from build123d import *

# Parameters (mm, degrees)
F0_W     = 50.8
F0_H     = 3.175
F1_DEPTH = 354.8
F2_R     = 2.6162
F2_R_2   = 3.175
F3_DEPTH = 3.176


with BuildPart() as f1:
    # F0 (on Front) → F1 (new body)
    with BuildSketch(Plane.XZ):
        Rectangle(F0_W, F0_H)
    extrude(amount=F1_DEPTH)

    # F2 (on face) → F3 (cut, through all)
    with BuildSketch(Plane.XY.offset(1.5875)):
        with Locations((0, -158.35)):
            Circle(F2_R)
        with Locations((0, -196.45)):
            Circle(F2_R)
        with Locations((-19.05, -329.4)):
            Circle(F2_R)
        with Locations((19.05, -329.4)):
            Circle(F2_R)
        with Locations((19.05, -25.4)):
            Circle(F2_R)
        with Locations((-19.05, -25.4)):
            Circle(F2_R)
        with Locations((-15.3416, -252.4)):
            Circle(F2_R)
        with Locations((15.3416, -252.4)):
            Circle(F2_R)
        with Locations((15.3416, -102.4)):
            Circle(F2_R)
        with Locations((-15.3416, -102.4)):
            Circle(F2_R)
        with Locations((0, -269.6254)):
            Circle(F2_R_2)
        with Locations((0, -85.1746)):
            Circle(F2_R_2)
    extrude(amount=-F3_DEPTH, mode=Mode.SUBTRACT)


solid = f1.part
Check sheet for the modelled part. Datum: model origin and axes. Units: mm. Coordinates: 2 decimals unless noted, no trailing zeros. Write item = value, one per line. Start each with the question number.
1. Material ranges on line 1 (Y direction, x = -19.05, z = -0.15); line 2 (Y direction, x = 0, z = 0.6); line 3 (Y direction, x = 1, z = -0.7), recorded low to high.
2. Draft check along Y on faces 1 (the flat face through (0, -175, 1.588)), 2 (the cylindrical face through (-0.688, -88.274, 0.022)). Enter one of: released by +Y, released by -Y, zero draft, split by the parting line, or undercut.
3. Section check A-A on z = -1. Give the number of separate pieces and of enclosed holes in the cut face, then the cut area to 3 significant figures.
4. Depth check by flat-ended pin: P1, Ø4.5, axis at x = 15.34, y = -102.4, coming from the -Z side. Enter the tip coordinate at first touch or a pass-through.
Responses:
q1.line_1 = -354.8 to -332.02, -326.78 to -28.02, -22.78 to 0
q1.line_2 = -354.8 to -272.8, -266.45 to -199.07, -193.83 to -160.97, -155.73 to -88.35, -82 to 0
q1.line_3 = -354.8 to -272.64, -266.61 to -198.87, -194.03 to -160.77, -155.93 to -88.19, -82.16 to 0
q2.face_1 = zero draft
q2.face_2 = undercut
q3.separate_pieces = 1
q3.enclosed_holes = 12
q3.area = 17,700 mm2
q4.P1 = through
